```python
from build123d import *

# Parameters (mm, degrees)
SKETCH2_R           = 10.01
BOSS_EXTRUDE1_DEPTH = 35
SKETCH3_R           = 15
BOSS_EXTRUDE2_DEPTH = 40
SKETCH4_R           = 12.5
BOSS_EXTRUDE3_DEPTH = 40


with BuildPart() as part:
    # Sketch2 → Boss-Extrude1 (new body)
    with BuildSketch(Plane.XY):
        Circle(SKETCH2_R)
    extrude(amount=-BOSS_EXTRUDE1_DEPTH)

    # Sketch3 → Boss-Extrude2 (add)
    with BuildSketch(Plane(origin=(0, 0, -35), x_dir=(-1, 0, 0), z_dir=(0, 0, -1))):
        Circle(SKETCH3_R)
    extrude(amount=BOSS_EXTRUDE2_DEPTH)

    # Sketch4 → Boss-Extrude3 (add)
    with BuildSketch(Plane(origin=(0, 0, -75), x_dir=(-1, 0, 0), z_dir=(0, 0, -1))):
        Circle(SKETCH4_R)
    extrude(amount=BOSS_EXTRUDE3_DEPTH)


solid = part.part
```
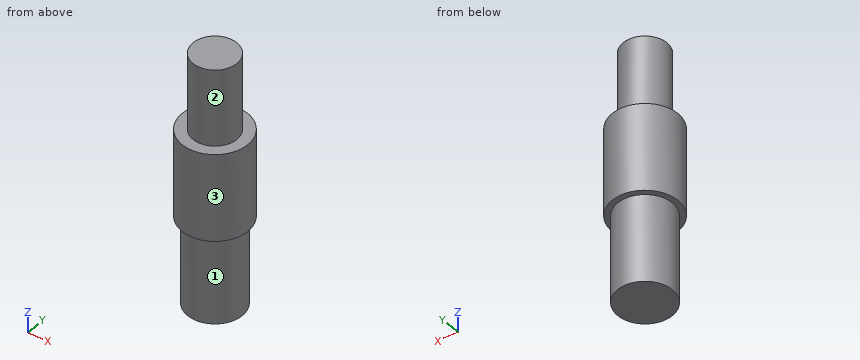
Design review of the part built by this model. Coordinates are the model's own, in mm. Face numbers are marked on the shaded views. A direction names the side the tool comes from. Give positions to 0.01 mm unless a question says otherwise; leave off trailing zeros. Order: outer loops, then holes, each group sorted by start corner. A loop starts at its lowest first (then second) coordinate and runs counter-clockwise, first axis right, second up. Notation, with made-up numbers: (15, 35) - (47, 35) arc R10 cw to (47, 52) - close; hole circle Ø6 at (57, 15). An arc over 180 degrees is marked (long way). Use a Markdown table: item, result. Add a question column.
(1) Add section C-C on z = -9.5. Give the boundary of the cut face in (x, y).
(2) Add section A-A on y = 0. Give the boundary of the cut face in (x, z).
(3) Machinability: for the marked faces 1, 2 and 3, which of the approach directions +Z, -Z, +X, -X, +Y, -Y give a long, thin tool a straight path to every point of the face, cutting with its end or side? Answer none if there is none.
(4) Add section D-D on z = -68. Give the boundary of the cut face in (x, y), then the cut area to 3 significant figures.
(5) Wall thickness on probe 1 along Y at (x, z) = (0.5, -103); probe 2 along Z at (x, y) = (1, -11); probe 3 along X at (y, z) = (0.75, -86): over which ranges is each line inside the solid? List them lowest first. Write a range as [from, to].
(6) Clearance check with flat-ended pins moving along their axes: P1, Ø8, axis at x = -10, z = -103, coming from the -Y side; P2, Ø12, axis at x = -12, z = -69, coming from the -Y side; P3, Ø4, axis at x = 6.5, z = -81, coming from the -Y side. State where each tip first meets the part, or that it passes through.
Report:
| question | item | result |
|---|---|---|
| 1 | outline | circle Ø20.02 at (0, 0) |
| 2 | outline | (-15, -75) - (-12.5, -75) - (-12.5, -115) - (12.5, -115) - (12.5, -75) - (15, -75) - (15, -35) - (10.01, -35) - (10.01, 0) - (-10.01, 0) - (-10.01, -35) - (-15, -35) - close |
| 3 | face 1 | -Z |
| 3 | face 2 | +Z |
| 3 | face 3 | +Z, -Z |
| 4 | outline | circle Ø30 at (0, 0) |
| 4 | area | 707 mm² |
| 5 | probe 1 | y = [-12.49, 12.49] |
| 5 | probe 2 | z = [-115, -35] |
| 5 | probe 3 | x = [-12.48, 12.48] |
| 6 | P1 | stops at y = -10.97 |
| 6 | P2 | stops at y = -13.75 |
| 6 | P3 | stops at y = -11.66 |
